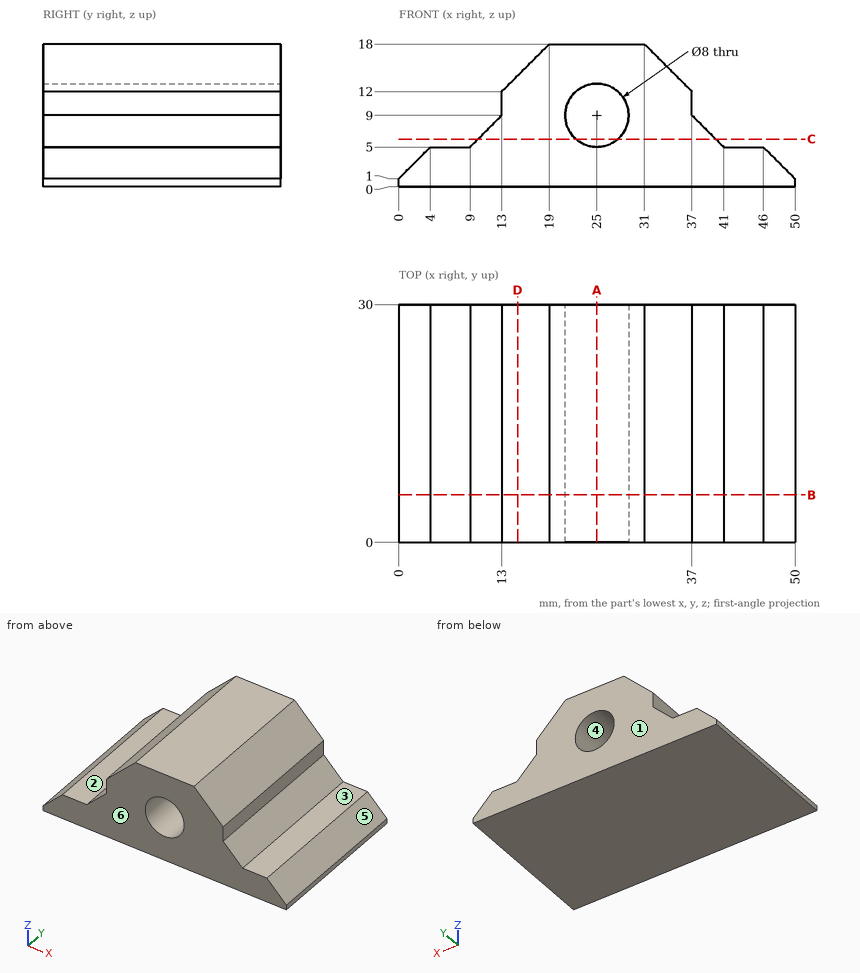
Geometry: see drawing. Coordinates: mm, zero at the bounding-box minimum. A direction names the side the tool comes from. Round coordinates to 2 decimals unless told otherwise and drop trailing zeros. Loops run counter-clockwise (first coordinate to the right, second up) from the corner with the lowest first, then second, coordinate; pieces in that order, holes last. Notation, with made-up numbers: M -28.75,79.5 L -24.75,79.5 A9 cw -24.75,85.5 Z; hole C -30.75,17.5 d3. An arc over 180 degrees is marked long. Use a Markdown table: item, result. Add a question column.
1. Section query D-D on x = 15. Return the cut outline in (y, z).
2. Section query B-B on y = 6. Return the cut outline in (x, z), then the cut area to 3 significant figures.
3. Section query A-A on x = 25. Return the cut outline in (y, z), then the cut area to 3 significant figures.
4. Mould query, pull axis X, two halves, no side actions, for the marked faces 4, 5 and 6. Classes: pulls with the +X half, pulls with the -X half, needs draft (parallel to the pull), parting line crosses it, or undercut.
5. Contact query for flat-ended pins moving along their axis: P1, Ø4, axis at x = 5.5, y = 21.5, coming from the +Z side; P2, Ø1, axis at y = 15.5, z = 8.5, coming from the -X side; P3, Ø3.5, axis at y = 14, z = 10.5, coming from the -X side. Output: stop coordinate, or through.
6. Section query C-C on z = 6. Return the cut outline in (x, y).
7. Reachability of the marked faces 1, 2 and 3 from +Z, -Z, +X, -X, +Y, -Y: full face, straight path, thin tool, end or side. Return the list, or none.
8. Line query: line 1 (Z direction, x = 25, y = 12.5); line 2 (X direction, y = 14.75, z = 9); line 3 (X direction, y = 11.5, z = 12.5). Output: solid intervals per line, ascending.
Reported:
| question | item | result |
|---|---|---|
| 1 | outline | M 0,0 L 30,0 L 30,14 L 0,14 Z |
| 2 | outline | M 0,0 L 50,0 L 50,1 L 46,5 L 41,5 L 37,9 L 37,12 L 31,18 L 19,18 L 13,12 L 13,9 L 9,5 L 4,5 L 0,1 Z; hole C 25,9 d8 |
| 2 | area | 476 mm² |
| 3 | outline | M 0,0 L 30,0 L 30,5 L 0,5 Z; M 0,13 L 30,13 L 30,18 L 0,18 Z |
| 3 | area | 300 mm² |
| 4 | face 4 | undercut |
| 4 | face 5 | pulls with the +X half |
| 4 | face 6 | needs draft |
| 5 | P1 | stops at z = 5 |
| 5 | P2 | stops at x = 12 |
| 5 | P3 | stops at x = 12.75 |
| 6 | outline | M 10,0 L 22.35,0 L 22.35,30 L 10,30 Z; M 27.65,0 L 40,0 L 40,30 L 27.65,30 Z |
| 7 | face 1 | +Z, -Z, +X, -X, +Y |
| 7 | face 2 | +Z, -X, +Y, -Y |
| 7 | face 3 | +Z, +X, +Y, -Y |
| 8 | line 1 | z = 0 to 5, 13 to 18 |
| 8 | line 2 | x = 13 to 21, 29 to 37 |
| 8 | line 3 | x = 13.5 to 23.06, 26.94 to 36.5 |
